Could you check a few things on this drawing? It's one solid part, dimensions in mm from its lowest x, y, z. A direction names the side the tool comes from. Give positions to 0.01 mm unless a question says otherwise; leave off trailing zeros. Loops run counter-clockwise (first coordinate to the right, second up) from the corner with the lowest first, then second, coordinate; pieces in that order, holes last. Notation, with made-up numbers: M 65.5,42.5 L 87.5,42.5 A15 ccw 87.5,62.5 Z; hole C 42.25,25.5 d5. An arc over 180 degrees is marked long. Answer as CSV lines item,"result". Start each with the question number.
Item 1: I want a section at D-D on x = 4. List the corners of the cut face in (y, z) for me (1 decimal).
Item 2: If we mould it in two halves opening along X, with no side actions, what happens to the marked faces 1, 2, 3 and 4? For each: released by +X, released by -X, zero draft, split by the parting line, or undercut.
Item 3: I want a section at A-A on x = 3. List the corners of the cut face in (y, z) for me, plus the area to 3 significant figures.
Item 4: Will these pins go through, and if not, where does the flat tip stop? P1, Ø3, axis at x = 3, y = 6.5, coming from the +Z side; P2, Ø1.6, axis at x = 3, z = 5, coming from the +Y side.
Item 5: I want a section at C-C on z = 4.2. List the corners of the cut face in (x, y) for me.
Item 6: If I drill on line 1 along Y through (x, z) = (3, 1.2); line 2 along Y through (x, z) = (3, 0.5); line 3 along Y through (x, z) = (4.05, 5.7), over which ranges is the centre line in solid material (lowest first)? Write a range as from..to.
Item 7: I want a section at B-B on y = 16. List the corners of the cut face in (x, z) for me.
Item 8: For the marked faces 5 and 6, which set-ups out of +Z, -Z, +X, -X, +Y, -Y let a thin tool reach every point of the face, with its end or its side?
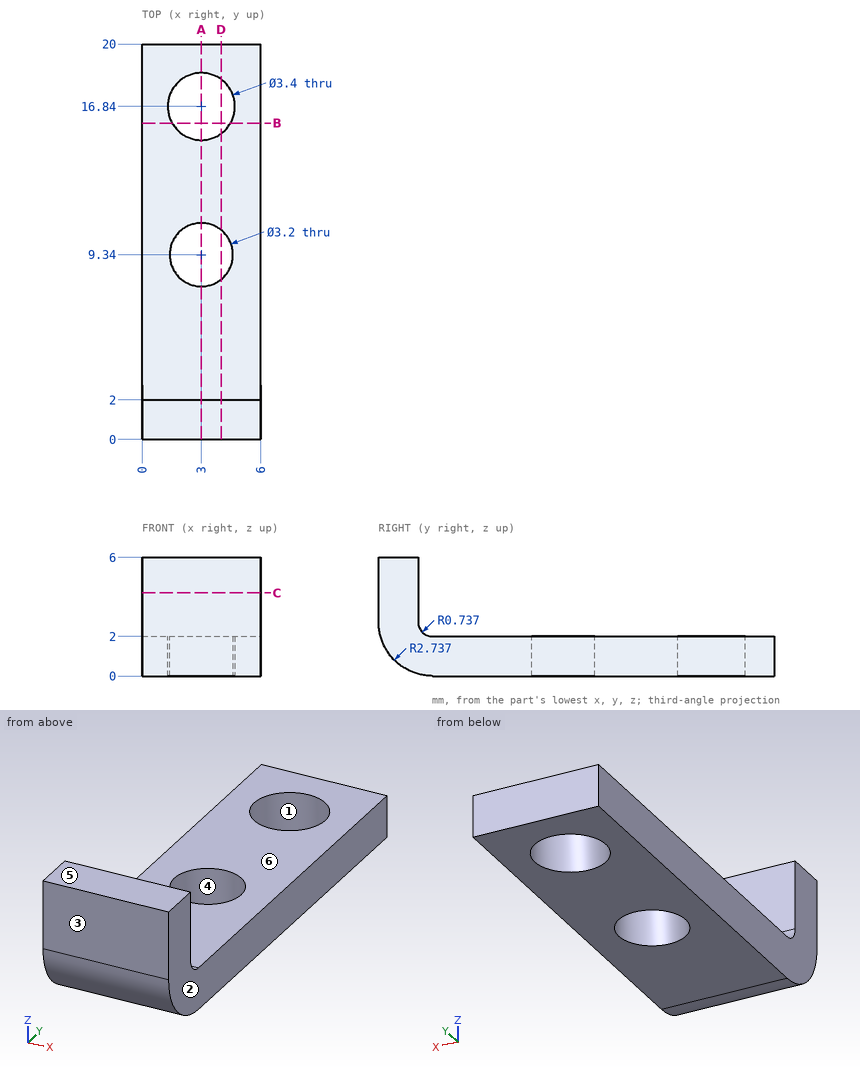
Result:
1,outline,"M 0,2.7 A2.7 ccw 2.7,0 L 8.1,0 L 8.1,2 L 2.7,2 A0.7 cw 2,2.7 L 2,6 L 0,6 Z; M 10.6,0 L 15.5,0 L 15.5,2 L 10.6,2 Z; M 18.2,0 L 20,0 L 20,2 L 18.2,2 Z"
2,face 1,"undercut"
2,face 2,"released by +X"
2,face 3,"zero draft"
2,face 4,"undercut"
3,outline,"M 0,2.74 A2.74 ccw 2.74,0 L 7.74,0 L 7.74,2 L 2.74,2 A0.74 cw 2,2.74 L 2,6 L 0,6 Z; M 10.94,0 L 15.14,0 L 15.14,2 L 10.94,2 Z; M 18.54,0 L 20,0 L 20,2 L 18.54,2 Z"
3,area,"33.3 mm^2"
4,P1,"z = 2"
4,P2,"y = 2"
5,outline,"M 0,0 L 6,0 L 6,2 L 0,2 Z"
6,line 1,"0.47..7.74, 10.94..15.14, 18.54..20"
6,line 2,"1.16..7.74, 10.94..15.14, 18.54..20"
6,line 3,"0..2"
7,outline,"M 0,0 L 1.52,0 L 1.52,2 L 0,2 Z; M 4.48,0 L 6,0 L 6,2 L 4.48,2 Z"
8,face 5,"+Z, +X, -X, +Y, -Y"
8,face 6,"+Z, +X, -X, +Y"
